Geometry: final body of the model. Coordinates: model frame, mm. A direction names the side the tool comes from. Round coordinates to 2 decimals unless told otherwise and drop trailing zeros. Write each loop counter-clockwise with the first axis right and the second up, starting at its lowest first coordinate (ties: lowest second). Pieces come first, ordered by that corner, then holes. Notation, with made-up numbers: M -39,-34.5 L -17,-34.5 A23 cw -17,-22.5 Z; hole C 71,52.25 d11. An arc over 180 degrees is marked long. Use one line per item in the form item = value. Start each with the question number.
Item 1: Section query B-B (y = 47). Return loops of the section in (x, z).
Item 2: Ray query, probe 1 along Y at (x, z) = (0, -5.25); probe 2 along Y at (x, z) = (-15.5, -4.5); probe 3 along X at (y, z) = (-11, -1.25). Return the intervals inside material, ascending.
Item 3: Reachability of faces 5 (the cylindrical face through (-80, 0.5, -5)), 6 (the flat face through (-32, 45, -2.5)), 7 (the flat face through (-12.398, 75.868, 6.093)), 8 (the cylindrical face through (71.831, -33.936, 12.839)) from +Z, -Z, +X, -X, +Y, -Y: full face, straight path, thin tool, end or side. Return the list, or none.
Item 4: Section query C-C (x = 29). Return loops of the section in (y, z).
Item 5: Pin query (flat end, axial travel): pin 1 Ø10.5 at (x, y) = (67, -53) entering from +Z; pin 2 Ø22 at (x, y) = (-45.5, 28.5) entering from +Z; pin 3 Ø4 at (x, z) = (54, 8.5) entering from +Y; pin 4 Ø12 at (y, z) = (-10, 10.5) entering from -X. Return the tip coordinate at first contact, or that it passes through.
Item 6: Pull-direction query (Y, two-part tool) for faces 1 (the flat face through (-55, 55, 20)), 2 (the flat face through (63.53, -51.57, 6.09)), 3 (the cylindrical face through (-19.704, 10.484, -4.965)), 4 (the cylindrical face through (19.723, 10.541, -4.965)); classes: pulls with the +Y half, pulls with the -Y half, needs draft (parallel to the pull), parting line crosses it, or undercut.
Item 7: Section query D-D (x = 2). Return loops of the section in (y, z) (3 decimals), and give its area (3 significant figures).
Item 8: Section query A-A (y = 0). Return loops of the section in (x, z).
from build123d import *

# Parameters (mm, degrees)
EXTRUDE_1_DEPTH                  = 20
EXTRUDE_1_DEPTH_BACK             = 7.5
EXTRUDE_3_DEPTH                  = 7.5
EXTRUDE_3_DEPTH_BACK             = 7.5
SKETCH_3_R                       = 21.5
SKETCH_4_R                       = 18.5
CUT_EXTRUDE_1_DEPTH              = 7.5
SKETCH_12_W                      = 5
SKETCH_12_H                      = 61
CUT_EXTRUDE_6_DEPTH              = 119.822346383
REVOLVE_START                    = -2.5
REVOLVE_3_DEPTH                  = 10
FILLET_1_R                       = 2
PATTERN_CIRCULAR_1_COUNT         = 2
PATTERN_CIRCULAR_1_ANGLE         = 90
FILLET_1_OF_PATTERN_CIRCULAR_1_R = 2
CUT_EXTRUDE_7_REACH              = 191.328
SKETCH_15_R                      = 4.2
CUT_EXTRUDE_8_REACH              = 191.328
SKETCH_16_R                      = 4.2
PATTERN_CIRCULAR_2_COUNT         = 3


# Read off the part's stored shape, not the designer's step: the revolve step
with BuildPart() as part:
    # Sketch 1 → Extrude 1 (new, two sides: drawn at the far end of the back side and taken through both)
    with BuildSketch(Plane.XY.offset(-EXTRUDE_1_DEPTH_BACK)):
        with BuildLine():
            Line((0, 82.5), (21.352571221, 79.688880669))
            ThreePointArc((21.352571221, 79.688880669), (71.447095812, 41.25), (79.688880669, -21.352571221))
            Line((79.688880669, -21.352571221), (71.447095812, -41.25))
            Line((71.447095812, -41.25), (58.336309448, -58.336309448))
            ThreePointArc((58.336309448, -58.336309448), (0, -82.5), (-58.336309448, -58.336309448))
            Line((-58.336309448, -58.336309448), (-71.447095812, -41.25))
            Line((-71.447095812, -41.25), (-79.688880669, -21.352571221))
            ThreePointArc((-79.688880669, -21.352571221), (-71.447095812, 41.25), (-21.352571221, 79.688880669))
            Line((-21.352571221, 79.688880669), (0, 82.5))
        make_face()
        with BuildLine():
            Line((0, 77.5), (20.058475995, 74.859251537))
            ThreePointArc((20.058475995, 74.859251537), (67.116968793, 38.75), (74.859251537, -20.058475995))
            Line((74.859251537, -20.058475995), (67.116968793, -38.75))
            Line((67.116968793, -38.75), (54.800775542, -54.800775542))
            ThreePointArc((54.800775542, -54.800775542), (0, -77.5), (-54.800775542, -54.800775542))
            Line((-54.800775542, -54.800775542), (-67.116968793, -38.75))
            Line((-67.116968793, -38.75), (-74.859251537, -20.058475995))
            ThreePointArc((-74.859251537, -20.058475995), (-67.116968793, 38.75), (-20.058475995, 74.859251537))
            Line((-20.058475995, 74.859251537), (0, 77.5))
        make_face(mode=Mode.SUBTRACT)
    extrude(amount=EXTRUDE_1_DEPTH + EXTRUDE_1_DEPTH_BACK)



with BuildPart() as body_2:
    # Sketch 3 → Extrude 3 (new, two sides: drawn at the far end of the back side and taken through both)
    with BuildSketch(Plane.XY.offset(-EXTRUDE_3_DEPTH_BACK)):
        Circle(SKETCH_3_R)
    extrude(amount=EXTRUDE_3_DEPTH + EXTRUDE_3_DEPTH_BACK)

    # Sketch 4 → Cut-Extrude 1 (cut)
    with BuildSketch(Plane(origin=(0, 0, -7.5), x_dir=(-1, 0, 0), z_dir=(0, 0, -1))):
        Circle(SKETCH_4_R)
    extrude(amount=-CUT_EXTRUDE_1_DEPTH, mode=Mode.SUBTRACT)


with BuildPart() as part_1:
    add(part.part)

    add(body_2.part)  # Revolve 2 merges body 2
    # Sketch 12 → Revolve 2 (revolve)
    with BuildSketch(Plane(origin=(0, 0, 0), x_dir=(0, 0, -1), z_dir=(1, 0, 0)), mode=Mode.PRIVATE) as revolve_2_sk:
        with Locations((5, 52)):
            Rectangle(SKETCH_12_W, SKETCH_12_H)
    revolve(revolve_2_sk.sketch.rotate(Axis((0, 0, 0), (0, 0, -1)), 90), axis=Axis((0, 0, 0), (0, 0, -1)))

    # Sketch 13 → Cut-Extrude 6 (cut, through all)
    with BuildSketch(Plane.XY.offset(-2.5)):
        with BuildLine():
            Line((-36.163690354, 62.637349082), (-12.157816416, 21.057955741))
            ThreePointArc((-12.157816416, 21.057955741), (-10.512484879, 19.713262861), (-8.389159771, 19.795757079))
            ThreePointArc((-8.389159771, 19.795757079), (0, 21.5), (8.389159771, 19.795757079))
            ThreePointArc((8.389159771, 19.795757079), (10.512484879, 19.713262861), (12.157816416, 21.057955741))
            Line((12.157816416, 21.057955741), (36.163690354, 62.637349082))
            ThreePointArc((36.163690354, 62.637349082), (36.615666268, 66.597311937), (34.028981496, 69.629580053))
            ThreePointArc((34.028981496, 69.629580053), (0, 77.5), (-34.028981496, 69.629580053))
            ThreePointArc((-34.028981496, 69.629580053), (-36.615666268, 66.597311937), (-36.163690354, 62.637349082))
        make_face()
        with BuildLine():
            Line((64.807406984, 37.416573868), (21.057955741, 12.157816416))
            ThreePointArc((21.057955741, 12.157816416), (19.713262861, 10.512484879), (19.795757079, 8.389159771))
            ThreePointArc((19.795757079, 8.389159771), (21.5, 0), (19.795757079, -8.389159771))
            ThreePointArc((19.795757079, -8.389159771), (19.713262861, -10.512484879), (21.057955741, -12.157816416))
            Line((21.057955741, -12.157816416), (64.807406984, -37.416573868))
            ThreePointArc((64.807406984, -37.416573868), (68.761859517, -37.870228599), (71.79456745, -35.292209972))
            ThreePointArc((71.79456745, -35.292209972), (80, 0), (71.79456745, 35.292209972))
            ThreePointArc((71.79456745, 35.292209972), (68.761859517, 37.870228599), (64.807406984, 37.416573868))
        make_face()
        with BuildLine():
            Line((37.416573868, -64.807406984), (12.157816416, -21.057955741))
            ThreePointArc((12.157816416, -21.057955741), (10.512484879, -19.713262861), (8.389159771, -19.795757079))
            ThreePointArc((8.389159771, -19.795757079), (0, -21.5), (-8.389159771, -19.795757079))
            ThreePointArc((-8.389159771, -19.795757079), (-10.512484879, -19.713262861), (-12.157816416, -21.057955741))
            Line((-12.157816416, -21.057955741), (-37.416573868, -64.807406984))
            ThreePointArc((-37.416573868, -64.807406984), (-37.870228599, -68.761859517), (-35.292209972, -71.79456745))
            ThreePointArc((-35.292209972, -71.79456745), (0, -80), (35.292209972, -71.79456745))
            ThreePointArc((35.292209972, -71.79456745), (37.870228599, -68.761859517), (37.416573868, -64.807406984))
        make_face()
        with BuildLine():
            Line((-64.807406984, -37.416573868), (-21.057955741, -12.157816416))
            ThreePointArc((-21.057955741, -12.157816416), (-19.713262861, -10.512484879), (-19.795757079, -8.389159771))
            ThreePointArc((-19.795757079, -8.389159771), (-21.5, 0), (-19.795757079, 8.389159771))
            ThreePointArc((-19.795757079, 8.389159771), (-19.713262861, 10.512484879), (-21.057955741, 12.157816416))
            Line((-21.057955741, 12.157816416), (-64.807406984, 37.416573868))
            ThreePointArc((-64.807406984, 37.416573868), (-68.761859517, 37.870228599), (-71.79456745, 35.292209972))
            ThreePointArc((-71.79456745, 35.292209972), (-80, 0), (-71.79456745, -35.292209972))
            ThreePointArc((-71.79456745, -35.292209972), (-68.761859517, -37.870228599), (-64.807406984, -37.416573868))
        make_face()
    extrude(amount=-CUT_EXTRUDE_6_DEPTH, mode=Mode.SUBTRACT)

    # Revolve 3 outline → Revolve 3 (add)
    with BuildSketch(Plane.XY.offset(REVOLVE_START)):
        with BuildLine():
            Line((52.854872905, 56.679911875), (14.662964741, 15.724104585))
            ThreePointArc((14.662964741, 15.724104585), (15.202795796, 15.202795796), (15.724104585, 14.662964741))
            Line((15.724104585, 14.662964741), (56.679911875, 52.854872905))
            ThreePointArc((56.679911875, 52.854872905), (54.800775542, 54.800775542), (52.854872905, 56.679911875))
        make_face()
    revolve_3 = extrude(amount=REVOLVE_3_DEPTH)

    # Fillet 1
    fillet_1_edges = [part_1.edges().sort_by_distance(p)[0] for p in [
        (52.854872905, 56.679911875, 2.5),
        (56.679911875, 52.854872905, 2.5),
    ]]
    fillet(fillet_1_edges, radius=FILLET_1_R)

    # Pattern Circular 1: Revolve 3 ×2 about axis
    pattern_circular_1_axis = Axis((0, 0, 0), (0, 0, 1))
    for i in range(1, PATTERN_CIRCULAR_1_COUNT):
        add(revolve_3.rotate(pattern_circular_1_axis, i * PATTERN_CIRCULAR_1_ANGLE / (PATTERN_CIRCULAR_1_COUNT - 1)))

    # Fillet 1 of Pattern Circular 1
    fillet_1_of_pattern_circular_1_edges = [part_1.edges().sort_by_distance(p)[0] for p in [
        (-56.679911875, 52.854872905, 2.5),
        (-52.854872905, 56.679911875, 2.5),
    ]]
    fillet(fillet_1_of_pattern_circular_1_edges, radius=FILLET_1_OF_PATTERN_CIRCULAR_1_R)

    # Sketch 15 → Cut-Extrude 7 (cut, up to next)
    with BuildSketch(Plane(origin=(10.67628561, 81.094440334, 0), x_dir=(0.991444861373809, -0.13052619222006237, 0), z_dir=(0.13052619222006237, 0.9914448613738092, 0)), mode=Mode.PRIVATE) as cut_extrude_7_sk1:
        with Locations(Location((-0.768410858, -10, 0), (0, 0, 180))):
            Circle(SKETCH_15_R)
    cut_extrude_7_tool1 = extrude(cut_extrude_7_sk1.sketch, amount=-CUT_EXTRUDE_7_REACH, mode=Mode.PRIVATE) & part_1.part
    cut_extrude_7 = cut_extrude_7_tool1.solids().sort_by_distance((9.914449, 81.194738, 10))[0]
    add(cut_extrude_7, mode=Mode.SUBTRACT)

    # Sketch 16 → Cut-Extrude 8 (cut, up to next)
    with BuildSketch(Plane(origin=(-10.67628561, 81.094440334, 0), x_dir=(0.991444861373809, 0.13052619222006237, 0), z_dir=(-0.13052619222006237, 0.9914448613738092, 0)), mode=Mode.PRIVATE) as cut_extrude_8_sk1:
        with Locations(Location((0.768410858, -10, 0), (0, 0, 180))):
            Circle(SKETCH_16_R)
    cut_extrude_8_tool1 = extrude(cut_extrude_8_sk1.sketch, amount=-CUT_EXTRUDE_8_REACH, mode=Mode.PRIVATE) & part_1.part
    cut_extrude_8 = cut_extrude_8_tool1.solids().sort_by_distance((-9.914449, 81.194738, 10))[0]
    add(cut_extrude_8, mode=Mode.SUBTRACT)

    # Pattern Circular 2: Cut-Extrude 7, Cut-Extrude 8 ×3 about axis
    pattern_circular_2_axis = Axis((0, 0, 0), (0, 0, 1))
    add([cut_extrude_7.rotate(pattern_circular_2_axis, i * 360 / PATTERN_CIRCULAR_2_COUNT) for i in range(1, PATTERN_CIRCULAR_2_COUNT)], mode=Mode.SUBTRACT)
    add([cut_extrude_8.rotate(pattern_circular_2_axis, i * 360 / PATTERN_CIRCULAR_2_COUNT) for i in range(1, PATTERN_CIRCULAR_2_COUNT)], mode=Mode.SUBTRACT)


solid = part_1.part
Working result:
q1.outline = M -67.8,-7.5 L -27.14,-7.5 L -27.14,-2.5 L -43.83,-2.5 L -43.83,7.5 L -50.4,7.5 L -50.4,-2.5 L -61.62,-2.5 L -61.62,20 L -67.8,20 Z; M 27.14,-7.5 L 67.8,-7.5 L 67.8,20 L 61.62,20 L 61.62,-2.5 L 50.4,-2.5 L 50.4,7.5 L 43.83,7.5 L 43.83,-2.5 L 27.14,-2.5 Z
q2.probe_1 = -82.5 to -80, -21.5 to -18.5, 18.5 to 21.5, 77.5 to 82.5
q2.probe_2 = -81.03 to -78.48, -26.85 to -10.1, 10.1 to 26.85, 75.93 to 81.03
q2.probe_3 = -81.76 to -76.72, -18.47 to -14.87, 14.87 to 18.47, 76.72 to 81.76
q3.face_5 = -Z
q3.face_6 = +Z
q3.face_7 = +Z, -Z
q3.face_8 = none
q4.outline = M -77.24,-7.5 L -74.56,-7.5 L -74.56,-2.5 L -71.87,-2.5 L -71.87,20 L -77.24,20 Z; M -50.23,-7.5 L -16.74,-7.5 L -16.74,-2.5 L -50.23,-2.5 Z; M 16.74,-7.5 L 50.23,-7.5 L 50.23,-2.5 L 31.1,-2.5 L 31.1,7.5 L 27.04,7.5 L 27.04,-2.5 L 16.74,-2.5 Z; M 71.87,-7.5 L 77.24,-7.5 L 77.24,20 L 71.87,20 Z
q5.pin_1 = 20
q5.pin_2 = 7.5
q5.pin_3 = 64.05
q5.pin_4 = -82.4
q6.face_1 = needs draft
q6.face_2 = pulls with the -Y half
q6.face_3 = undercut
q6.face_4 = undercut
q7.outline = M -82.476,-7.5 L -79.975,-7.5 L -79.975,-2.5 L -77.474,-2.5 L -77.474,20 L -82.476,20 Z; M -21.407,-7.5 L -18.392,-7.5 L -18.392,0 L 18.392,0 L 18.392,-7.5 L 21.407,-7.5 L 21.407,7.5 L -21.407,7.5 Z; M 77.237,-2.5 L 77.474,-2.5 L 77.474,-7.5 L 82.476,-7.5 L 82.476,-2.5 L 82.237,-2.5 L 82.237,20 L 77.237,20 Z
q7.area = 629 mm²
q8.outline = M -82.5,-7.5 L -80,-7.5 L -80,-2.5 L -77.5,-2.5 L -77.5,20 L -82.5,20 Z; M -21.5,-7.5 L -18.5,-7.5 L -18.5,0 L 18.5,0 L 18.5,-7.5 L 21.5,-7.5 L 21.5,7.5 L -21.5,7.5 Z; M 77.5,-2.5 L 80,-2.5 L 80,-7.5 L 82.5,-7.5 L 82.5,20 L 77.5,20 Z
